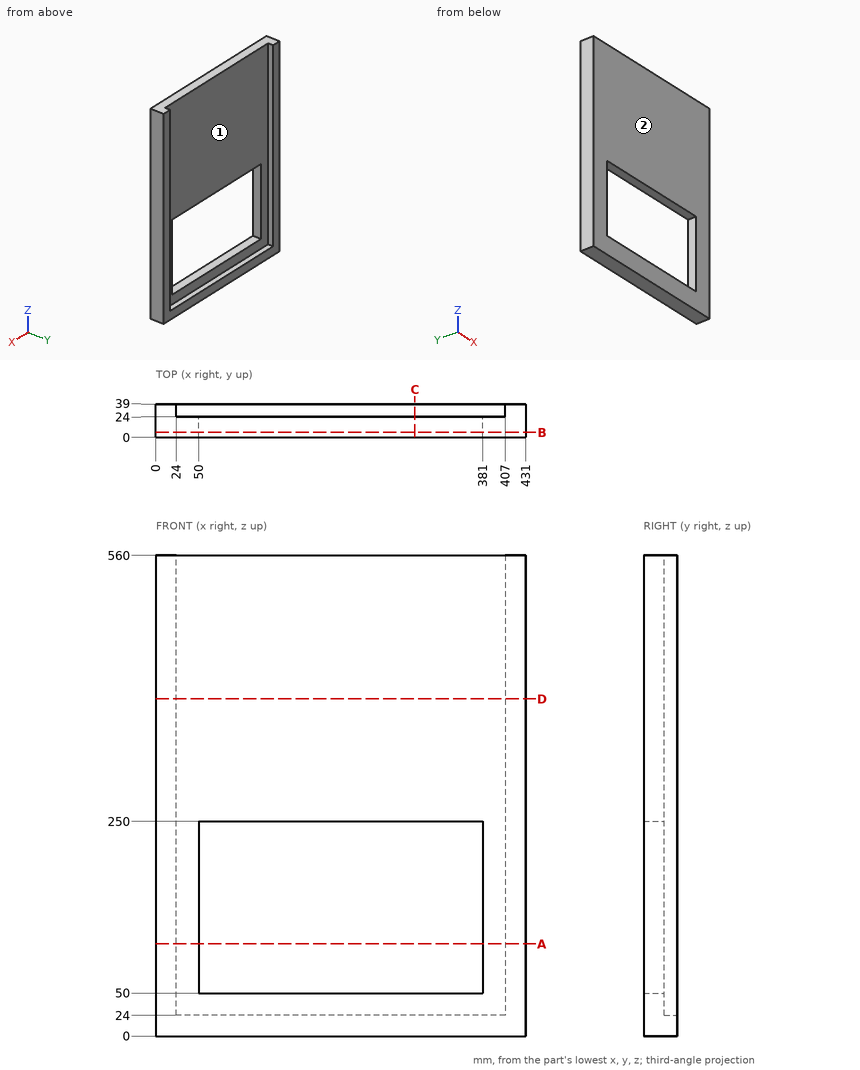
Part print with two shaded views. Sizes in mm from the minimum x, y, z corner. Coordinates: 2 decimals unless noted, no trailing zeros. Write each loop counter-clockwise with the first axis right and the second up, starting at its lowest first coordinate (ties: lowest second). Pieces come first, ordered by that corner, then holes. Notation, with made-up numbers: (-34.5, 30) - (7.5, 30) arc R24 cw to (7.5, 69) - close; hole circle Ø8 at (49, 19.5). An arc over 180 degrees is marked (long way). One line per item, written item: value. Start each with the question number.
1. Slice it at D-D (z = 393). Write the cut outline in (x, y), plus the area to 3 significant figures.
2. Probe line 1 (Z direction, x = 318.5, y = 20); line 2 (X direction, y = 34, z = 494); line 3 (Y direction, x = 32.5, z = 98). List the from-to ranges inside material, lowest first. Write a range as from..to.
3. Slice it at B-B (y = 6). Write the cut outline in (x, z), plus the area to 3 significant figures.
4. Flat gauge pins, fed straight in: pin 1 (1 mm diameter, centred on x = 256, y = 31.5, fed in from +Z); pin 2 (12 mm diameter, centred on x = 136, y = 18, fed in from -Z). Where does each tip first touch, or does it go through?
5. Mould opens along X. For the marked faces 1 and 2 say: released by +X, released by -X, zero draft, split by the parting line, or undercut.
6. Slice it at C-C (x = 302). Write the cut outline in (y, z), plus the area to 3 significant figures.
7. Slice it at A-A (z = 107.5). Write the cut outline in (x, y).
Answers below:
1. outline: (0, 0) - (431, 0) - (431, 39) - (407, 39) - (407, 24) - (24, 24) - (24, 39) - (0, 39) - close
1. area: 11,100 mm^2
2. line 1: z = 0..50, 250..560
2. line 2: x = 0..24, 407..431
2. line 3: y = 0..24
3. outline: (0, 0) - (431, 0) - (431, 560) - (0, 560) - close; hole (50, 50) - (381, 50) - (381, 250) - (50, 250) - close
3. area: 175,000 mm^2
4. pin 1: stops at z = 24
4. pin 2: stops at z = 0
5. face 1: undercut
5. face 2: zero draft
6. outline: (0, 0) - (39, 0) - (39, 24) - (24, 24) - (24, 50) - (0, 50) - close; (0, 250) - (24, 250) - (24, 560) - (0, 560) - close
6. area: 9,000 mm^2
7. outline: (0, 0) - (50, 0) - (50, 24) - (24, 24) - (24, 39) - (0, 39) - close; (381, 0) - (431, 0) - (431, 39) - (407, 39) - (407, 24) - (381, 24) - close
